Part model, mm, in its own coordinate system. A direction names the side the tool comes from. Coordinates: 2 decimals unless noted, no trailing zeros. Order: outer loops, then holes, each group sorted by start corner. A loop starts at its lowest first (then second) coordinate and runs counter-clockwise, first axis right, second up.
Autodesk Inventor part; units mm, degrees
ref_plane "YZ Plane" through (0, 0, 0) normal (1, 0, 0) x (0, 1, 0)
ref_plane "XZ Plane" through (0, 0, 0) normal (0, 1, 0) x (-1, 0, 0)
ref_plane "XY Plane" through (0, 0, 0) normal (0, 0, 1) x (1, 0, 0)
sketch "Esboço1" plane through (0, 0, 0) normal (0, 0, 1) x (1, 0, 0)
  circle A0 centre (0, 0) radius 25.5
  dimension "d0" = 51
extrude "Extrusão1" add sketch "Esboço1" along normal blind 3
sketch "Esboço2" plane through (0, 0, 3) normal (0, 0, 1) x (1, 0, 0)
  circle A0 centre (0, 0) radius 17.5
  circle A1 centre (-0.0486, 21.9399) radius 1.5
  line L0 (-0.0486, 17.4999) -> (-0.0486, -17.4999)
  dimension "d3" = 35
  dimension "d4" = 21.94
  dimension "d5" = 3
extrude "Extrusão2" add sketch "Esboço2" along normal blind 12 contours A0 L0 | L0 A0
sketch "Esboço3" plane through (0, 0, 3) normal (0, 0, 1) x (1, 0, 0)
  circle A0 centre (0, 0) radius 17.5
  point P0 (0, 21.94)
  point P1 (-19.0006, -10.97)
  point P2 (19.0006, -10.97)
  dimension "d8" = 21.94
  dimension "d11" = 360
hole "Furo1" at (0, 21.94, 3) at (-19.0006, -10.97, 3) at (19.0006, -10.97, 3) direction (0, 0, -1) diameter 3 end through all
properties part number "Motor mesh" material "Alumínio 6061"
(1) Tool access for faces 1 (the face through (0, 0, 15)), 2 (the face through (-6, -17, 3)): list every direction of +Z, -Z, +X, -X, +Y, -Y with a clear straight run to the whole face (end or side of a thin tool).
(2) Slice it at B-B, the plane y = -10.97. Give the cut face in (x, z), then the cut area to 3 significant figures.
(3) Probe line 1 (Y direction, x = 0, z = 1.45); line 2 (X direction, y = -10.97, z = 1.1); line 3 (Z direction, x = -18, y = -16.5). List the from-to ranges inside material, lowest first.
(4) Slice it at C-C, the plane y = 21.94. Give the cut face in (x, z), then the cut area to 3 significant figures.
(5) Drop flat-ended pins along their axis: pin 1 (2.5 mm diameter, centred on x = 0, y = 21.94, fed in from -Z); pin 2 (8 mm diameter, centred on x = -15, z = 11.5, fed in from -Y); pin 3 (3 mm diameter, centred on x = -15, z = 3, fed in from -Y); pin 4 (5 mm diameter, centred on x = -19, y = -10.97, fed in from +Z). Give the stop position or say it passes through.
(6) Slice it at D-D, the plane z = 10.75. Give the cut face in (x, y).
(7) Slice it at A-A, the plane x = 0. Give the cut face in (y, z).
Here are the results:
1. face 1: +Z, +X, -X, +Y, -Y
1. face 2: +Z
2. outline: (-23.02, 0) - (-20.5, 0) - (-20.5, 3) - (-23.02, 3) - close; (-17.5, 0) - (17.5, 0) - (17.5, 3) - (13.63, 3) - (13.63, 15) - (-13.63, 15) - (-13.63, 3) - (-17.5, 3) - close; (20.5, 0) - (23.02, 0) - (23.02, 3) - (20.5, 3) - close
2. area: 447 mm2
3. line 1: y = -25.5 to 20.44, 23.44 to 25.5
3. line 2: x = -23.02 to -20.5, -17.5 to 17.5, 20.5 to 23.02
3. line 3: z = 0 to 3
4. outline: (-13, 0) - (-1.5, 0) - (-1.5, 3) - (-13, 3) - close; (1.5, 0) - (13, 0) - (13, 3) - (1.5, 3) - close
4. area: 69.0 mm2
5. pin 1: passes through
5. pin 2: stops at y = -13.61
5. pin 3: stops at y = -21.63
5. pin 4: stops at z = 3
6. outline: circle Ø35 at (0, 0)
7. outline: (-25.5, 0) - (20.44, 0) - (20.44, 3) - (17.5, 3) - (17.5, 15) - (-17.5, 15) - (-17.5, 3) - (-25.5, 3) - close; (23.44, 0) - (25.5, 0) - (25.5, 3) - (23.44, 3) - close
